Verification items for the finished model (mm, model axes). A direction names the side the tool comes from. Round coordinates to 2 decimals unless told otherwise and drop trailing zeros. Order: outer loops, then holes, each group sorted by start corner. A loop starts at its lowest first (then second) coordinate and runs counter-clockwise, first axis right, second up.
```python
from build123d import *

# Parameters (mm, degrees)
SKETCH1_R           = 5
BOSS_EXTRUDE1_DEPTH = 18
SKETCH2_R           = 8
BOSS_EXTRUDE2_DEPTH = 3
BOSS_EXTRUDE2_TAPER = 60
CUT_EXTRUDE1_DEPTH  = 1
FILLET1_R           = 0.5


with BuildPart() as part:
    # Sketch1 → Boss-Extrude1 (new body)
    with BuildSketch(Plane(origin=(0, 0, 0), x_dir=(0, 0, -1), z_dir=(1, 0, 0))):
        Circle(SKETCH1_R)
    extrude(amount=BOSS_EXTRUDE1_DEPTH)

    # Sketch2 → Boss-Extrude2 (add)
    with BuildSketch(Plane.ZY):
        Circle(SKETCH2_R)
    extrude(amount=BOSS_EXTRUDE2_DEPTH, taper=BOSS_EXTRUDE2_TAPER)

    # Sketch4 → Cut-Extrude1 (cut)
    with BuildSketch(Plane.ZY.offset(3)):
        Polygon((2.340832904, 0), (1.170416452, 2.027220761), (-1.170416452, 2.027220761), (-2.340832904, 0), (-1.170416452, -2.027220761), (1.170416452, -2.027220761), align=None)
    extrude(amount=-CUT_EXTRUDE1_DEPTH, mode=Mode.SUBTRACT)

    # Fillet1
    fillet1_edges = [part.edges().sort_by_distance(p)[0] for p in [
        (-2, -1.01361038, 1.755624678),
        (-2, -2.027220761, 0),
        (-2, -1.01361038, -1.755624678),
        (-2, 1.01361038, -1.755624678),
        (-2, 2.027220761, 0),
        (-2, 1.01361038, 1.755624678),
    ]]
    fillet(fillet1_edges, radius=FILLET1_R)


solid = part.part
```
1) Tool access check on faces 4 (the flat face through (-3, -1, -2)), 5 (the cylindrical face through (-2.15, 0.93, -1.64)), 6 (the cylindrical face through (8.87, -4.88, 1.08)). Record the directions out of +Z, -Z, +X, -X, +Y, -Y that give a thin tool (end or side, any length) a straight path to the whole face; none if there is none.
2) Sectioned sample at A-A on z = 0. Record the cut outline in (x, y), then the cut area to 3 significant figures.
3) Scan lines: probe 1 along Y at (x, z) = (3.25, -0.25); probe 2 along X at (y, z) = (4.5, 0.5); probe 3 along Z at (x, y) = (3, 3). Record each from-to range of solid material in increasing order.
4) Go/stop test with flat-tipped pins: pin 1 Ø4 at (x, y) = (6, -6) entering from -Z; pin 2 Ø1.5 at (x, y) = (3, 5) entering from -Z; pin 3 Ø5 at (x, z) = (3, -5) entering from -Y. Record where each tip stops, or that it passes through.
5) Draft check along Z on faces 1 (the conical face through (-2.85, -1.86, -2.43)), 2 (the flat face through (18, 0, 0)), 3 (the cylindrical face through (-2.15, -0.96, -1.62)). Enter one of: released by +Z, released by -Z, zero draft, split by the parting line, or undercut.
6) Sectioned sample at B-B on x = 6. Record the cut outline in (y, z).
Returned:
1. face 4: +Z, -Z, -X, +Y, -Y
1. face 5: -X
1. face 6: +X
2. outline: (-3, -2.8) - (0, -8) - (0, -5) - (18, -5) - (18, 5) - (0, 5) - (0, 8) - (-3, 2.8) - (-3, 2.03) - (-2.5, 2.03) arc R0.5 cw to (-2, 1.53) - (-2, -1.53) arc R0.5 cw to (-2.5, -2.03) - (-3, -2.03) - close
2. area: 208 mm2
3. probe 1: y = -4.99 to 4.99
3. probe 2: x = -2 to 18
3. probe 3: z = -4 to 4
4. pin 1: stops at z = -3
4. pin 2: stops at z = -2.63
4. pin 3: stops at y = -4.33
5. face 1: split by the parting line
5. face 2: zero draft
5. face 3: undercut
6. outline: circle Ø10 at (0, 0)
